Geometry: final body of the model. Coordinates: model frame, mm. A direction names the side the tool comes from. Give positions to 0.01 mm unless a question says otherwise; leave off trailing zeros. Write each loop counter-clockwise with the first axis right and the second up, starting at its lowest first coordinate (ties: lowest second). Pieces come first, ordered by that corner, then holes. Notation, with made-up numbers: (-32.5, 16.5) -> (-20.5, 16.5) arc R11 ccw to (-20.5, 33.5) -> close; hole circle Ø11 at (37.25, 34.25). An arc over 180 degrees is marked (long way). Answer as a JSON object with one key per item and string values.
from build123d import *

# Parameters (mm, degrees)
SKETCH_1_W             = 23
SKETCH_1_H             = 17
EXTRUDE_1_DEPTH        = 6.5
SKETCH_2_W             = 20
SKETCH_2_H             = 15.5
CUT_EXTRUDE_1_DEPTH    = 5
SKETCH_3_W             = 23
SKETCH_3_H             = 1.5
EXTRUDE_2_DEPTH        = 12.6
FILLET_1_R             = 3
EXTRUDE_3_DEPTH        = 3
HOLE_WIZARD_M3_1_D     = 3.2
EXTRUDE_START          = -11.5
EXTRUDE_6_DEPTH        = 1.5
CUT_EXTRUDE_2534_REACH = 21.059
SKETCH_10_W            = 6
SKETCH_10_H            = 3.5
SKETCH_11_W            = 1.5
SKETCH_11_H            = 9
EXTRUDE_10_DEPTH       = 12.910593501
SKETCH_12_W            = 1
SKETCH_12_H            = 9
EXTRUDE_11_DEPTH       = 14
HOLE_WIZARD_M3_2_D     = 3.2


# Read off the part's stored shape, not the designer's step: 凸台-拉伸6
with BuildPart() as part:
    # 草图1 → 凸台-拉伸1 (new body)
    with BuildSketch(Plane.XY):
        Rectangle(SKETCH_1_W, SKETCH_1_H)
    extrude(amount=EXTRUDE_1_DEPTH)

    # 草图2 → 切除-拉伸1 (cut)
    with BuildSketch(Plane.XY.offset(6.5)):
        with Locations((0, -0.75)):
            Rectangle(SKETCH_2_W, SKETCH_2_H)
    extrude(amount=-CUT_EXTRUDE_1_DEPTH, mode=Mode.SUBTRACT)

    # 草图3 → 凸台-拉伸2 (add)
    with BuildSketch(Plane(origin=(0, 0, 0), x_dir=(-1, 0, 0), z_dir=(0, 0, -1))):
        with Locations((0, -7.75)):
            Rectangle(SKETCH_3_W, SKETCH_3_H)
    extrude(amount=EXTRUDE_2_DEPTH)

    # 圆角1
    fillet_1_edges = [part.edges().sort_by_distance(p)[0] for p in [
        (11.5, -7.75, -12.6),
        (-11.5, -7.75, -12.6),
    ]]
    fillet(fillet_1_edges, radius=FILLET_1_R)

    # 草图4 → 凸台-拉伸3 (add)
    with BuildSketch(Plane(origin=(0, -7, 0), x_dir=(1, 0, 0), z_dir=(0, 1, 0))):
        Polygon((5.080682369, 6.4), (2.540341184, 10.8), (-2.540341184, 10.8), (-5.080682369, 6.4), (-2.540341184, 2), (2.540341184, 2), align=None)
        Polygon((3.348631561, 6.4), (1.674315781, 9.3), (-1.674315781, 9.3), (-3.348631561, 6.4), (-1.674315781, 3.5), (1.674315781, 3.5), align=None, mode=Mode.SUBTRACT)
    extrude(amount=EXTRUDE_3_DEPTH)

    # M3 间隙孔1 (through all)
    with Locations(Plane(origin=(0, -7, 0), x_dir=(1, 0, 0), z_dir=(0, 1, 0))):
        with Locations((0, 6.4)):
            Hole(HOLE_WIZARD_M3_1_D / 2)

    # 凸台-拉伸6 outline → 凸台-拉伸6 (add)
    with BuildSketch(Plane.YZ.offset(EXTRUDE_START)):
        Polygon((-7, 0), (-7, -10.266991259), (3.266991259, 0), align=None)
    extrude(amount=EXTRUDE_6_DEPTH)

    # 草图10 → Cut-Extrude 2534 (cut, up to next)
    with BuildSketch(Plane(origin=(0, 0, 0), x_dir=(-1, 0, 0), z_dir=(0, 0, -1)), mode=Mode.PRIVATE) as cut_extrude_2534_sk1:
        with Locations((0, -2.75)):
            Rectangle(SKETCH_10_W, SKETCH_10_H)
    cut_extrude_2534_tool1 = extrude(cut_extrude_2534_sk1.sketch, amount=-CUT_EXTRUDE_2534_REACH, mode=Mode.PRIVATE) & part.part
    add(cut_extrude_2534_tool1.solids().sort_by_distance((0, -2.75, 0))[0], mode=Mode.SUBTRACT)

    # 草图11 → 凸台-拉伸10 (add)
    with BuildSketch(Plane(origin=(0, 0, 0), x_dir=(-1, 0, 0), z_dir=(0, 0, -1))):
        with Locations((-10.75, 3.3)):
            Rectangle(SKETCH_11_W, SKETCH_11_H)
    extrude(amount=EXTRUDE_10_DEPTH)

    # 草图12 → 凸台-拉伸11 (add)
    with BuildSketch(Plane(origin=(11.5, 0, 0), x_dir=(0, 0, -1), z_dir=(1, 0, 0))):
        with Locations((12.410593501, 3.3)):
            Rectangle(SKETCH_12_W, SKETCH_12_H)
    extrude(amount=EXTRUDE_11_DEPTH)

    # M3 间隙孔2 (through all)
    with Locations(Plane.XY.offset(-11.910593501)):
        with Locations((18.5, 3.3)):
            Hole(HOLE_WIZARD_M3_2_D / 2)


solid = part.part
Q1. Cut plane A-A (x = 0). Return the cut outline in (y, z).
Values:
{"outline": "(-8.5, -12.6) -> (-7, -12.6) -> (-7, -10.8) -> (-4, -10.8) -> (-4, -9.3) -> (-7, -9.3) -> (-7, -8) -> (-8.5, -8) -> close; (-8.5, -4.8) -> (-7, -4.8) -> (-7, -3.5) -> (-4, -3.5) -> (-4, -2) -> (-7, -2) -> (-7, 0) -> (-4.5, 0) -> (-4.5, 1.5) -> (-8.5, 1.5) -> close; (-1, 0) -> (8.5, 0) -> (8.5, 6.5) -> (7, 6.5) -> (7, 1.5) -> (-1, 1.5) -> close"}
Q2. Cut plane D-D (y = -6). Return the cut outline in (x, z), and give its area (3 significant figures).
Values:
{"outline": "(-11.5, -9.27) -> (-10, -9.27) -> (-10, 0) -> (11.5, 0) -> (11.5, 6.5) -> (10, 6.5) -> (10, 1.5) -> (-10, 1.5) -> (-10, 6.5) -> (-11.5, 6.5) -> close; (-5.08, -6.4) -> (-2.54, -10.8) -> (2.54, -10.8) -> (5.08, -6.4) -> (2.54, -2) -> (-2.54, -2) -> close; hole (-3.35, -6.4) -> (-1.67, -9.3) -> (1.67, -9.3) -> (3.35, -6.4) -> (1.67, -3.5) -> (-1.67, -3.5) -> close", "area": "101 mm²"}
Q3. Set-up query: faces 4 (the flat face through (-3.793, -5.521, -8.631)), 5 (the flat face through (10, -1, 4)), 6 (the flat face through (0, -4.5, 1)), 7 (the flat face through (3.793, -5.521, -4.169)), 8 (the flat face through (2, -7, -6)). Return all of +Z, -Z, +X, -X, +Y, -Y with unobstructed straight access to the full face (end or side cutting, diameter ignored); none if empty.
Values:
{"face 4": "-Z, +Y", "face 5": "+Z, -Y", "face 6": "+Z", "face 7": "+X, +Y", "face 8": "+Y"}
Q4. Cut plane C-C (z = -8.5). Return the cut outline in (x, y).
Values:
{"outline": "(-11.5, -8.5) -> (11.5, -8.5) -> (11.5, -7) -> (3.87, -7) -> (3.87, -4) -> (2.14, -4) -> (2.14, -7) -> (-2.14, -7) -> (-2.14, -4) -> (-3.87, -4) -> (-3.87, -7) -> (-10, -7) -> (-10, -5.23) -> (-11.5, -5.23) -> close; (10, -1.2) -> (11.5, -1.2) -> (11.5, 7.8) -> (10, 7.8) -> close"}
Q5. Mould query, pull axis X, two halves, no side actions, for faces 1 (the flat face through (-0.1, -0.6, 1.5)), 2 (the flat face through (3.83, -5.52, -8.57)), 3 (the flat face through (0, -8.5, -3)). Classes: pulls with the +X half, pulls with the -X half, needs draft (parallel to the pull), parting line crosses it, or undercut.
Values:
{"face 1": "undercut", "face 2": "pulls with the +X half", "face 3": "needs draft"}
Q6. Cut plane B-B (x = 18.5). Return the cut outline in (y, z).
Values:
{"outline": "(-1.2, -12.91) -> (1.7, -12.91) -> (1.7, -11.91) -> (-1.2, -11.91) -> close; (4.9, -12.91) -> (7.8, -12.91) -> (7.8, -11.91) -> (4.9, -11.91) -> close"}
Q7. Material intervals for L1, parallel to Y at x = 18.5, z = -12.2; L2, parallel to Z at x = 0, y = -7.95; L3, parallel to X at y = 1.5, z = 3.5, sorted ascending. Write a range as from..to.
Values:
{"L1": "-1.2..1.7, 4.9..7.8", "L2": "-12.6..-8, -4.8..1.5", "L3": "-11.5..-10, 10..11.5"}
Q8. First-contact query: P1, Ø8, axis at y = -5.5, z = -7.5, coming from the +X side; P2, Ø0.9, axis at x = 0.5, y = -5, coming from the -Z side; P3, Ø7, axis at x = 20, y = 5, coming from the +Z side. Flat tips, straight axial feed; report the tip coordinate or a pass-through.
Values:
{"P1": "x = 11.5", "P2": "z = -10.8", "P3": "z = -11.91"}
